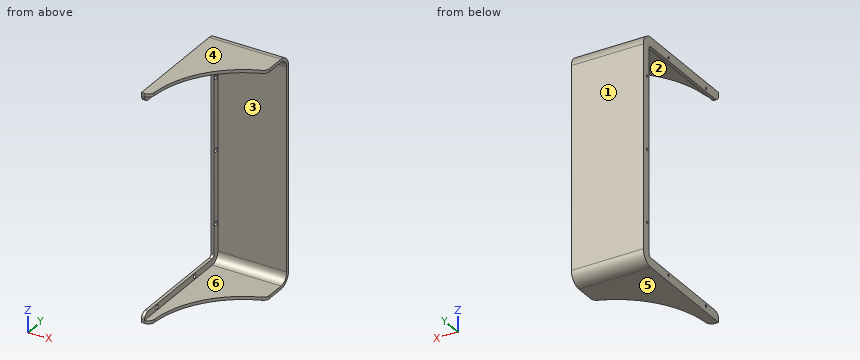
from build123d import *

# Parameters (mm, degrees)
BOSS_EXTRUDE1_DEPTH = 70
BOSS_EXTRUDE2_DEPTH = 3
SKETCH2_R           = 90
CUT_EXTRUDE1_DEPTH  = 239.537208838
FILLET2_R           = 9
FILLET3_R           = 3
FILLET4_R           = 12
FILLET5_R           = 6
SKETCH3_R           = 2
CUT_EXTRUDE2_DEPTH  = 2
SKETCH4_R           = 1.1
CUT_EXTRUDE3_DEPTH  = 3


with BuildPart() as part:
    # Sketch1 → Boss-Extrude1 (new body)
    with BuildSketch(Plane(origin=(0, 0, 0), x_dir=(0, 0, -1), z_dir=(1, 0, 0))):
        Polygon((-107, -60), (-107, 57), (107, 57), (107, -60), (110, -60), (110, 60), (-110, 60), (-110, -60), align=None)
    extrude(amount=BOSS_EXTRUDE1_DEPTH)

    # Sketch1<3> → Boss-Extrude2 (add)
    with BuildSketch(Plane(origin=(0, 0, 0), x_dir=(0, 0, -1), z_dir=(1, 0, 0))):
        Polygon((107, 57), (-107, 57), (-107, -60), (-101, -60), (-101, 51), (101, 51), (101, -60), (107, -60), align=None)
    extrude(amount=BOSS_EXTRUDE2_DEPTH)

    # Sketch2 → Cut-Extrude1 (cut, through all)
    with BuildSketch(Plane.XY.offset(110)):
        with Locations((99, -60)):
            Circle(SKETCH2_R)
    extrude(amount=-CUT_EXTRUDE1_DEPTH, mode=Mode.SUBTRACT)

    # Fillet2
    fillet2_edges = [part.edges().sort_by_distance(p)[0] for p in [
        (36.5, 57, -107),
        (36.5, 57, 107),
    ]]
    fillet(fillet2_edges, radius=FILLET2_R)

    # Fillet3
    fillet3_edges = [part.edges().sort_by_distance(p)[0] for p in [
        (1.5, 51, -101),
        (1.5, 51, 101),
    ]]
    fillet(fillet3_edges, radius=FILLET3_R)

    # Fillet4
    fillet4_edges = [part.edges().sort_by_distance(p)[0] for p in [
        (35, 60, 110),
        (35, 60, -110),
    ]]
    fillet(fillet4_edges, radius=FILLET4_R)

    # Fillet5
    fillet5_edges = [part.edges().sort_by_distance(p)[0] for p in [
        (1.5, -60, 101),
        (9, -60, 108.5),
        (1.5, -60, -101),
        (9, -60, -108.5),
        (70, 25.199765258, -108.5),
        (70, 25.199765258, 108.5),
    ]]
    fillet(fillet5_edges, radius=FILLET5_R)

    # Sketch3 → Cut-Extrude2 (cut)
    with BuildSketch(Plane(origin=(3, 0, 0), x_dir=(0, 0, -1), z_dir=(1, 0, 0))):
        with Locations((-104, -40)):
            Circle(SKETCH3_R)
        with Locations((-104, 20)):
            Circle(SKETCH3_R)
        with Locations((-70, 54)):
            Circle(SKETCH3_R)
        with Locations((0, 54)):
            Circle(SKETCH3_R)
        with Locations((70, 54)):
            Circle(SKETCH3_R)
        with Locations((104, 20)):
            Circle(SKETCH3_R)
        with Locations((104, -40)):
            Circle(SKETCH3_R)
    extrude(amount=-CUT_EXTRUDE2_DEPTH, mode=Mode.SUBTRACT)

    # Sketch4 → Cut-Extrude3 (cut)
    with BuildSketch(Plane(origin=(3, 0, 0), x_dir=(0, 0, -1), z_dir=(1, 0, 0))):
        with Locations((-104, -40)):
            Circle(SKETCH4_R)
        with Locations((-104, 20)):
            Circle(SKETCH4_R)
        with Locations((-70, 54)):
            Circle(SKETCH4_R)
        with Locations((0, 54)):
            Circle(SKETCH4_R)
        with Locations((70, 54)):
            Circle(SKETCH4_R)
        with Locations((104, 20)):
            Circle(SKETCH4_R)
        with Locations((104, -40)):
            Circle(SKETCH4_R)
    extrude(amount=-CUT_EXTRUDE3_DEPTH, mode=Mode.SUBTRACT)


solid = part.part
Can you work these out from the model? Positions are in its coordinate system, mm. Face numbers are marked on the shaded views. A direction names the side the tool comes from. Coordinates: 2 decimals unless noted, no trailing zeros. Write each loop counter-clockwise with the first axis right and the second up, starting at its lowest first coordinate (ties: lowest second). Pieces come first, ordered by that corner, then holes. Notation, with made-up numbers: (52, 43) - (97, 43) arc R8 cw to (97, 58) - close; hole circle Ø6 at (-31, 27). An arc over 180 degrees is marked (long way). Return JSON: item names as keys, results as strings. Group by question number.
Item 1: If we section it at A-A (y = 12): Write out the boundary of the cut face in (x, z).
Item 2: Please list where these lines run through material, in increasing order: probe 1 along Z at (x, y) = (33, 46); probe 2 along Y at (x, z) = (1.4, -104); probe 3 along Y at (x, z) = (0.4, -70).
Item 3: Which directions (+Z, -Z, +X, -X, +Y, -Y) give clear straight access to the entire face, cutting with the end or side of a thin tool? Please do the marked faces 5 and 6.
Item 4: We'd pull the mould along Z, two halves only. Please class the marked faces 1, 2, 3 and 4: pulls with the +Z half, pulls with the -Z half, needs draft (parallel to the pull), parting line crosses it, or undercut.
Item 5: If we section it at B-B (z = -18.5): Write out the boundary of the cut face in (x, y), then the cut area to 3 significant figures.
Item 6: I'm going to push flat-ended pins straight in: pin 1 Ø3.5 at (x, z) = (1.5, 25.5) entering from -Y; pin 2 Ø4.5 at (y, z) = (20.5, -104.5) entering from +X; pin 3 Ø1.3 at (y, z) = (-40, -104) entering from +X; pin 4 Ø1.2 at (y, z) = (-40.5, 103.5) entering from +X. Where does each tip first touch, or does it pass through?
Item 7: If we section it at C-C (x = 27): Write out the boundary of the cut face in (y, z).
Item 8: If we section it at D-D (y = 44): Write out the boundary of the cut face in (x, z).
Return value:
{
 "1": {"outline": "(0, -110) - (45, -110) - (45, -107) - (3, -107) - (3, -101) - (0, -101) - close; (0, 101) - (3, 101) - (3, 107) - (45, 107) - (45, 110) - (0, 110) - close"},
 "2": {"probe 1": "z = -110 to -107, 107 to 110", "probe 2": "y = -59.2 to -42, -38 to 18, 22 to 58.39", "probe 3": "y = 51 to 52.9, 55.1 to 60"},
 "3": {"face 5": "-Z, +X, -X, +Y, -Y", "face 6": "+X, -Y"},
 "4": {"face 1": "needs draft", "face 2": "undercut", "face 3": "undercut", "face 4": "pulls with the +Z half"},
 "5": {"outline": "(0, 51) - (3, 51) - (3, 57) - (70, 57) - (70, 60) - (0, 60) - close", "area": "228 mm^2"},
 "6": {"pin 1": "stops at y = 51", "pin 2": "stops at x = 3", "pin 3": "passes through", "pin 4": "stops at x = 1"},
 "7": {"outline": "(-6, -110) - (48, -110) arc R12 ccw to (60, -98) - (60, 98) arc R12 ccw to (48, 110) - (-6, 110) - (-6, 107) - (48, 107) arc R9 cw to (57, 98) - (57, -98) arc R9 cw to (48, -107) - (-6, -107) - close"},
 "8": {"outline": "(0, -110) - (70, -110) - (70, -107) - (3, -107) - (3, -101) - (0, -101) - close; (0, 101) - (3, 101) - (3, 107) - (70, 107) - (70, 110) - (0, 110) - close"}
}
